```python
from build123d import *

# Parameters (mm, degrees)
SKETCH1_W                 = 282.575
SKETCH1_H                 = 384.175
CELL_BODY_DEPTH           = 277.495
SKETCH5_W                 = 120.65
SKETCH5_H                 = 121.92
SEE_THROUGH_HOLE_DEPTH    = 282.575
SKETCH6_R                 = 12.7
CHIMNEY_DEPTH             = 63.5
SKETCH9_R                 = 10.16
CHIMNEY_COUNTERBORE_DEPTH = 50.8
SKETCH10_R                = 5.566584011
CHIMNEY_HOLE_DEPTH        = 98.806


with BuildPart() as part:
    # Sketch1 → Cell body (new body)
    with BuildSketch(Plane.XY):
        Rectangle(SKETCH1_W, SKETCH1_H)
    extrude(amount=-CELL_BODY_DEPTH)

    # Sketch5 → see-through hole (cut)
    with BuildSketch(Plane.XY):
        with Locations((0, 47.989561969)):
            Rectangle(SKETCH5_W, SKETCH5_H)
    extrude(amount=-SEE_THROUGH_HOLE_DEPTH, mode=Mode.SUBTRACT)

    # Sketch6 → Chimney (add)
    with BuildSketch(Plane(origin=(0, 192.0875, 0), x_dir=(1, 0, 0), z_dir=(0, 1, 0))):
        with Locations(Location((0, 141.2875, 0), (0, 0, 270))):
            Circle(SKETCH6_R)
    extrude(amount=CHIMNEY_DEPTH)

    # Sketch9 → Chimney counterbore (cut)
    with BuildSketch(Plane(origin=(0, 255.5875, 0), x_dir=(1, 0, 0), z_dir=(0, 1, 0))):
        with Locations(Location((0, 141.2875, 0), (0, 0, 270))):
            Circle(SKETCH9_R)
    extrude(amount=-CHIMNEY_COUNTERBORE_DEPTH, mode=Mode.SUBTRACT)

    # Sketch10 → Chimney hole (cut)
    with BuildSketch(Plane(origin=(0, 204.7875, 0), x_dir=(1, 0, 0), z_dir=(0, 1, 0))):
        with Locations(Location((0, 141.2875, 0), (0, 0, 270))):
            Circle(SKETCH10_R)
    extrude(amount=-CHIMNEY_HOLE_DEPTH, mode=Mode.SUBTRACT)


solid = part.part
```
The listing builds one solid part. Answer for the finished solid, in the listing's coordinates (mm). A direction names the side the tool comes from. Give positions to 0.01 mm unless a question says otherwise; leave off trailing zeros. Order: outer loops, then holes, each group sorted by start corner. A loop starts at its lowest first (then second) coordinate and runs counter-clockwise, first axis right, second up. Notation, with made-up numbers: (59.5, -15.5) - (105.5, -15.5) arc R11 cw to (105.5, 3.5) - close; hole circle Ø10 at (-32, -18). An arc over 180 degrees is marked (long way). Answer in a Markdown table with one row per item. Add a question column.
Q1. Given P1, Ø8, axis at x = -112, y = 3, coming from the +Z side, flat-ended and moving along its own axis, determine where the tip first touches the part or whether it passes through.
Q2. Find the intervals of material crossed by line 1 along Y through (x, z) = (46.5, -191.5); line 2 along X through (y, z) = (5.5, -135) (1 decimal); line 3 along Y through (x, z) = (101.5, -219), in increasing order. Write a range as [from, to].
Q3. The part is cut by section C-C (z = -201.5). Determine the outline of the cut face in (x, y) (1 decimal), then the cut area to 3 significant figures.
Q4. The part is cut by section D-D (y = 213). Determine the outline of the cut face in (x, z), then the cut area to 3 significant figures.
Q5. The part is cut by section A-A (y = 53). Determine the outline of the cut face in (x, z) (1 decimal), then the cut area to 3 significant figures.
Q6. For a pull along Z with two mould halves and no side action, classify faces 4 (the flat face through (141.288, -3, -137)), 5 (the cylindrical face through (8.58, 223.39, -150.65)), 6 (the cylindrical face through (0.447, 230.543, -151.438)) as released by +Z, released by -Z, zero draft, split by the parting line, or undercut.
Q7. The part is cut by section B-B (x = 0). Determine the outline of the cut face in (y, z) (1 decimal), then the cut area to 3 significant figures.
Q8. Which of the six approach directions +Z, -Z, +X, -X, +Y, -Y give full straight-line access (tool end or side, diameter ignored) to faces 1 (the flat face through (9, 255.588, -147)), 2 (the flat face through (-4, 204.788, -137)), 3 (the flat face through (-60.325, 47, -137))?
Determined:
| question | item | result |
|---|---|---|
| 1 | P1 | stops at z = 0 |
| 2 | line 1 | y = [-192.09, -12.97], [108.95, 192.09] |
| 2 | line 2 | x = [-141.3, -60.3], [60.3, 141.3] |
| 2 | line 3 | y = [-192.09, 192.09] |
| 3 | outline | (-141.3, -192.1) - (141.3, -192.1) - (141.3, 192.1) - (-141.3, 192.1) - close; hole (-60.3, -13) - (60.3, -13) - (60.3, 108.9) - (-60.3, 108.9) - close |
| 3 | area | 93,800 mm² |
| 4 | outline | circle Ø25.4 at (0, -141.29); hole circle Ø20.32 at (0, -141.29) |
| 4 | area | 182 mm² |
| 5 | outline | (-141.3, -277.5) - (-60.3, -277.5) - (-60.3, 0) - (-141.3, 0) - close; (60.3, -277.5) - (141.3, -277.5) - (141.3, 0) - (60.3, 0) - close |
| 5 | area | 44,900 mm² |
| 6 | face 4 | zero draft |
| 6 | face 5 | split by the parting line |
| 6 | face 6 | undercut |
| 7 | outline | (-192.1, -277.5) - (-13, -277.5) - (-13, 0) - (-192.1, 0) - close; (108.9, -277.5) - (192.1, -277.5) - (192.1, -154) - (255.6, -154) - (255.6, -151.4) - (204.8, -151.4) - (204.8, -146.9) - (108.9, -146.9) - close; (108.9, -135.7) - (204.8, -135.7) - (204.8, -131.1) - (255.6, -131.1) - (255.6, -128.6) - (192.1, -128.6) - (192.1, 0) - (108.9, 0) - close |
| 7 | area | 72,300 mm² |
| 8 | face 1 | +Z, -Z, +X, -X, +Y |
| 8 | face 2 | +Y |
| 8 | face 3 | +Z, -Z |
